Source: three-view drawing plus pictorial views. Frame: mm from the lowest corner of the part. Round coordinates to 2 decimals unless told otherwise and drop trailing zeros. Loops run counter-clockwise (first coordinate to the right, second up) from the corner with the lowest first, then second, coordinate; pieces in that order, holes last. Notation, with made-up numbers: (-3.5, 42.25) -> (41.5, 42.25) arc R21 cw to (41.5, 74.25) -> close; hole circle Ø4 at (79.5, -27). An arc over 180 degrees is marked (long way). Put each result on its own line as item: value. Start each with the question number.
1. Cut plane B-B (z = 6.5). Return the cut outline in (x, y), then the cut area to 3 significant figures.
2. Cut plane C-C (x = 36). Return the cut outline in (y, z) (1 decimal).
3. Contact query for flat-ended pins moving along their axis: pin 1 (10 mm diameter, centred on y = 12, z = 46.5, fed in from +X) (1 decimal); pin 2 (1 mm diameter, centred on x = 32, y = 9.5, fed in from +Z); pin 3 (1.5 mm diameter, centred on y = 9.5, z = 12, fed in from +X). Output: stop coordinate, or through.
4. Material intervals for L1, parallel to Z at x = 7, y = 16.5 (1 decimal); L2, parallel to Z at x = 18.5, y = 18.5; L3, parallel to X at y = 19.75, z = 33, sorted ascending.
5. Cut plane A-A (y = 7.25). Return the cut outline in (x, z) (1 decimal), then the cut area to 3 significant figures.
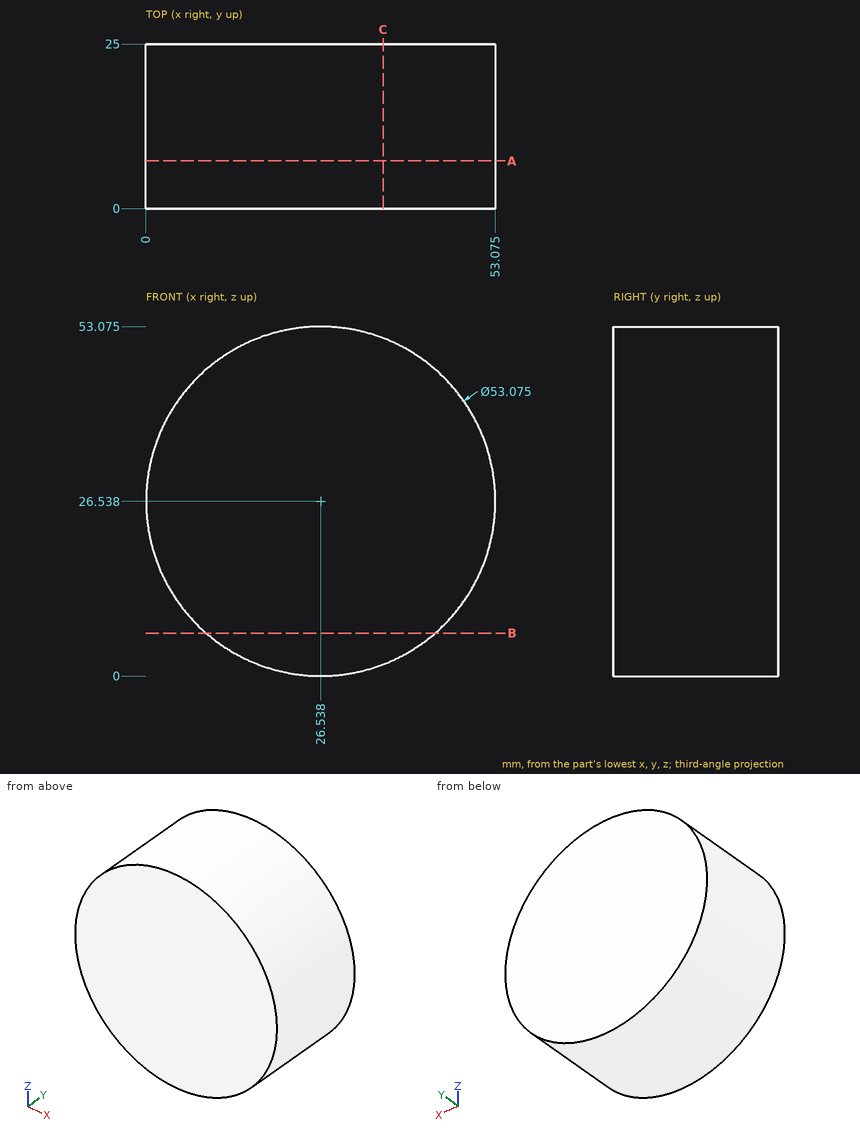
Solution:
1. outline: (9.14, 0) -> (43.94, 0) -> (43.94, 25) -> (9.14, 25) -> close
1. area: 870 mm^2
2. outline: (0, 1.7) -> (25, 1.7) -> (25, 51.3) -> (0, 51.3) -> close
3. pin 1: stops at x = 48.5
3. pin 2: stops at z = 52.61
3. pin 3: stops at x = 49.21
4. L1: z = 8.6 to 44.5
4. L2: z = 1.25 to 51.83
4. L3: x = 0.8 to 52.28
5. outline: circle Ø53.1 at (26.5, 26.5)
5. area: 2,210 mm^2
